Verification items for the finished model (mm, model axes). Face numbers are marked on the shaded views. A direction names the side the tool comes from. Give positions to 0.01 mm unless a question says otherwise; leave off trailing zeros. Write each loop counter-clockwise with the first axis right and the second up, starting at its lowest first coordinate (ties: lowest second). Pieces come first, ordered by that corner, then holes. Notation, with made-up numbers: (56.5, 81.25) - (68.5, 81.25) arc R7 cw to (68.5, 93.25) - close; hole circle Ø6 at (11, 82.5). An arc over 180 degrees is marked (long way). Answer as a JSON object with one key per item and string values. Group by question number.
Item 1: Tool access check on the marked faces 5, 6, 7 and 8. Record the directions out of +Z, -Z, +X, -X, +Y, -Y that give a thin tool (end or side, any length) a straight path to the whole face; none if there is none.
Item 2: Draft check along Z on the marked faces 1, 2, 3 and 4. Enter one of: +Z half, -Z half, draft (parallel to the pull), parting line (faces both ways), or undercut.
Item 3: Go/stop test with flat-tipped pins: pin 1 (5.5 mm diameter, centred on x = 4.98, y = 5.02, fed in from +Z); pin 2 (1.5 mm diameter, centred on y = 1, z = 3.5, fed in from -X). Record where each tip stops, or that it passes through.
Item 4: Scan lines: line 1 along Z through (x, y) = (5.5, 1.25); line 2 along Z through (x, y) = (3, 4.25). Record each from-to range of solid material in increasing order. Write a range as [from, to].
Item 5: Sectioned sample at B-B, the plane z = 9.5. Record the boundary of the cut face in (x, y).
```python
from build123d import *

# Parameters (mm, degrees)
BOX_W           = 10
BOX_H           = 10
BOX_DEPTH       = 10
SKETCH_R        = 3.031933
SKETCH_R_2      = 1.466661
PAD_DEPTH       = 0.25
SKETCH001_R     = 2.993457
SKETCH001_R_2   = 1.531672
PAD001_DEPTH    = 0.25
SKETCH002_W     = 2.724157
SKETCH002_H     = 6.368804
POCKET_DEPTH    = 0.1
POCKET001_DEPTH = 0.1
SKETCH004_R     = 3.031957
PAD002_DEPTH    = 1.2
CHAMFER_SIZE    = 0.5
SKETCH005_R     = 3.00622
POCKET002_DEPTH = 1


with BuildPart() as part:
    # Box → Box (new body)
    with BuildSketch(Plane.XY):
        with Locations((5, 5)):
            Rectangle(BOX_W, BOX_H)
    extrude(amount=BOX_DEPTH)

    # Sketch → Pad (new body)
    with BuildSketch(Plane(origin=(0, 0, 0), x_dir=(0, -1, 0), z_dir=(-1, 0, 0))):
        with Locations((-4.966039, 4.966038)):
            Circle(SKETCH_R)
        with Locations((-4.966039, 4.966038)):
            Circle(SKETCH_R_2, mode=Mode.SUBTRACT)
    extrude(amount=PAD_DEPTH)

    # Sketch001 → Pad001 (new body)
    with BuildSketch(Plane.YZ.offset(10)):
        with Locations((5, 5.033968)):
            Circle(SKETCH001_R)
        with Locations((5, 5.033968)):
            Circle(SKETCH001_R_2, mode=Mode.SUBTRACT)
    extrude(amount=PAD001_DEPTH)

    # Sketch002 → Pocket (cut)
    with BuildSketch(Plane.XZ):
        Polygon((1.199389, 9.955067), (1.199389, 1.230168), (8.845252, 1.230168), (8.845252, 9.984818), (7.653271, 9.984818), (7.653271, 2.423196), (2.426231, 2.423196), (2.426231, 9.955067), align=None)
        with Locations((5.033784, 6.775435)):
            Rectangle(SKETCH002_W, SKETCH002_H)
    extrude(amount=-POCKET_DEPTH, mode=Mode.SUBTRACT)

    # Sketch003 → Pocket001 (cut)
    with BuildSketch(Plane(origin=(0, 10, 0), x_dir=(-1, 0, 0), z_dir=(0, 1, 0))):
        Polygon((-1.217365, 9.989383), (-8.787637, 9.989383), (-8.787637, 2.392008), (-7.501711, 2.392008), (-7.501711, 8.826966), (-2.287892, 8.826966), (-2.287892, 2.401849), (-1.217365, 2.401849), align=None)
        Polygon((-9.019255, 0), (-0.963062, 0), (-0.963062, 1.125345), (-3.413274, 1.125345), (-3.413274, 7.666882), (-6.368116, 7.666882), (-6.368116, 1.205942), (-9.019255, 1.205942), align=None)
    extrude(amount=-POCKET001_DEPTH, mode=Mode.SUBTRACT)

    # Sketch004 → Pad002 (new body)
    with BuildSketch(Plane(origin=(0, 0, 0), x_dir=(1, 0, 0), z_dir=(0, 0, -1))):
        with Locations((5.012299, -4.970473)):
            Circle(SKETCH004_R)
    extrude(amount=PAD002_DEPTH)

    # Chamfer
    chamfer_edges = [part.edges().sort_by_distance(p)[0] for p in [
        (1.980342, 4.970473, -1.2),
    ]]
    chamfer(chamfer_edges, length=CHAMFER_SIZE)

    # Sketch005 → Pocket002 (cut)
    with BuildSketch(Plane.XY.offset(10)):
        with Locations((4.981398, 5.022974)):
            Circle(SKETCH005_R)
    extrude(amount=-POCKET002_DEPTH, mode=Mode.SUBTRACT)


solid = part.part
```
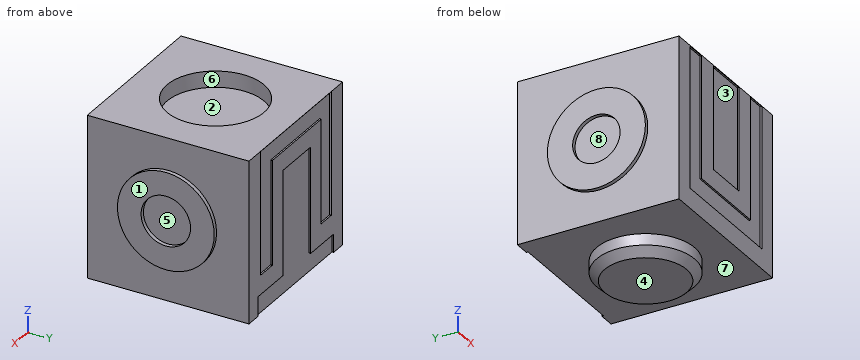
Geometry check:
{
 "1": {"face 5": "+X", "face 6": "+Z", "face 7": "-Z", "face 8": "-X"},
 "2": {"face 1": "draft", "face 2": "+Z half", "face 3": "undercut", "face 4": "-Z half"},
 "3": {"pin 1": "z = 9", "pin 2": "x = 0"},
 "4": {"line 1": "[0, 10]", "line 2": "[-1.2, 9]"},
 "5": {"outline": "(0, 0) - (1.2, 0) - (1.2, 0.1) - (2.43, 0.1) - (2.43, 0) - (3.67, 0) - (3.67, 0.1) - (6.4, 0.1) - (6.4, 0) - (7.65, 0) - (7.65, 0.1) - (8.85, 0.1) - (8.85, 0) - (10, 0) - (10, 10) - (8.79, 10) - (8.79, 9.9) - (1.22, 9.9) - (1.22, 10) - (0, 10) - close; hole circle Ø6.01 at (4.98, 5.02)"}
}
